```python
from build123d import *

# Parameters (mm, degrees)
BOSS_EXTRUDE1_DEPTH            = 6.35
F_1_16_0_0625_DIAMETER_HOLE1_D = 1.5875


# Read off the part's stored shape, not the designer's step: Boss-Extrude1
with BuildPart() as part:
    # Boss-Extrude1 outline → Boss-Extrude1 (new body)
    with BuildSketch(Plane.XY):
        Polygon((43.641394901, 180), (43.641394901, 190), (49.991394901, 190), (49.991394901, 200), (30, 200), (30, 206.35), (20, 206.35), (20, 200), (6.35, 200), (6.35, 190), (0, 190), (0, 180), (6.35, 180), (6.35, 170), (0, 170), (0, 160), (6.35, 160), (6.35, 150), (0, 150), (0, 140), (6.35, 140), (6.35, 130), (0, 130), (0, 120), (6.35, 120), (6.35, 110), (0, 110), (0, 100), (6.35, 100), (6.35, 90), (0, 90), (0, 80), (6.35, 80), (6.35, 70), (0, 70), (0, 60), (6.35, 60), (6.35, 50), (0, 50), (0, 40), (6.35, 40), (6.35, 30), (0, 30), (0, 20), (6.35, 20), (6.35, 10), (0, 10), (0, 0), (20, 0), (20, -6.35), (30, -6.35), (30, 0.011738555), (43.641394901, 0), (43.641394901, 10), (50, 10), (50, 20), (43.641394901, 20), (43.641394901, 30), (50, 30), (50, 40), (43.641394901, 40), (43.641394901, 50), (50, 50), (50, 60), (43.641394901, 60), (43.641394901, 70), (50, 70), (50, 80), (43.641394901, 80), (43.641394901, 90), (50, 90), (50, 100), (43.641394901, 100), (43.641394901, 110), (50, 110), (50, 120), (43.641394901, 120), (43.641394901, 130), (50, 130), (50, 140), (43.641394901, 140), (43.641394901, 150), (50, 150), (50, 160), (43.641394901, 160), (43.641394901, 170), (50, 170), (50, 180), align=None)
    extrude(amount=BOSS_EXTRUDE1_DEPTH)

    # 1/16 (0.0625) Diameter Hole1 (through all)
    with Locations(Plane.XY.offset(6.35)):
        with Locations((6.35, 190), (6.35, 180), (6.35, -2541.231306405), (20, 200), (30, 200), (43.641394901, 190), (43.641394901, 180), (43.641394901, 170), (43.641394901, 160), (43.641394901, 150), (6.35, 150), (6.35, 160), (6.35, 140), (6.35, -2581.231306405), (6.35, 120), (6.35, 110), (6.35, 100), (6.35, 90), (6.35, 80), (6.35, 70), (6.35, 60), (6.35, 50), (6.35, 40), (6.35, 30), (6.35, 20), (6.35, 10), (43.641394901, 140), (43.641394901, 130), (43.641394901, 120), (43.641394901, 110), (43.641394901, 100), (43.641394901, 90), (43.641394901, 80), (43.641394901, 70), (43.641394901, 60), (43.641394901, 50), (43.641394901, 40), (43.641394901, 30), (43.641394901, 20), (43.641394901, 10), (30, 0.011738555), (20, 0)):
            Hole(F_1_16_0_0625_DIAMETER_HOLE1_D / 2)


solid = part.part
```
The model under review builds one solid part; all positions refer to its coordinate system, in mm. A direction names the side the tool comes from. Round coordinates to 2 decimals unless told otherwise and drop trailing zeros. Loops run counter-clockwise (first coordinate to the right, second up) from the corner with the lowest first, then second, coordinate; pieces in that order, holes last.
1) The part is to be moulded in two halves that separate along Y. For faces 1 (the face through (3, 160, 3)), 2 (the face through (13, 200, 3)), 3 (the face through (6.35, 195, 3)), 4 (the face through (43.641, 185, 3)), say which applies: pulls with the +Y half, pulls with the -Y half, needs draft (parallel to the pull), parting line crosses it, or undercut.
Values follow:
face 1: undercut
face 2: pulls with the +Y half
face 3: needs draft
face 4: undercut
2) Clearance check with flat-ended pins moving along their axes: P1, Ø1.5, axis at x = 41, z = 3, coming from the +Y side; P2, Ø2, axis at x = 33, z = 1.5, coming from the -Y side; P3, Ø3, axis at x = 2.5, z = 3.5, coming from the +Y side. State where each tip first meets the part, or that it passes through.
Values follow:
P1: stops at y = 200
P2: stops at y = 0.01
P3: stops at y = 190
3) Tool access review of faces 5 (the face through (43.641, 125, 3)), 6 (the face through (50, 55, 3)), 7 (the face through (3, 150, 3)): name each direction out of +Z, -Z, +X, -X, +Y, -Y from which nothing blocks a thin tool from reaching the whole face with its end or side.
Values follow:
face 5: +Z, -Z, +X
face 6: +Z, -Z, +X, +Y, -Y
face 7: +Z, -Z, -X
4) Consider section B-B on x = 34.5. State the section outline as (y, z) points.
Values follow:
outline: (0.01, 0) - (200, 0) - (200, 6.35) - (0.01, 6.35) - close
5) Wall thickness on line 1 along X through (y, z) = (88, 1.25); line 2 along X through (y, z) = (92, 4); line 3 along Y through (x, z) = (20.5, 5.5): over which ranges is each line inside the solid? List them lowest first.
Values follow:
line 1: x = 0 to 43.64
line 2: x = 6.35 to 50
line 3: y = -6.35 to -0.62, 0.62 to 199.38, 200.62 to 206.35
6) Consider section A-A on x = 13.5. State the section outline as (y, z) points.
Values follow:
outline: (0, 0) - (200, 0) - (200, 6.35) - (0, 6.35) - close
